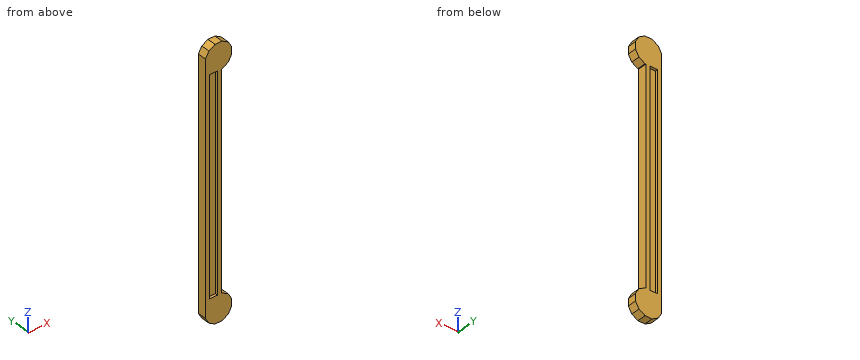
from build123d import *

# Parameters (mm, degrees)
BOSS_EXTRUDE1_DEPTH = 22
CUT_EXTRUDE1_DEPTH  = 635.24127901
SKETCH3_W           = 20
SKETCH3_H           = 534
CUT_EXTRUDE2_DEPTH  = 6.5
SKETCH4_W           = 20
SKETCH4_H           = 534
CUT_EXTRUDE3_DEPTH  = 6.5


with BuildPart() as part:
    # Sketch1 → Boss-Extrude1 (new body)
    with BuildSketch(Plane(origin=(0, 11, 0), x_dir=(1, 0, 0), z_dir=(0, 1, 0))):
        Polygon((24.15767665, 24.15767665), (8.84232335, 33), (-8.84232335, 33), (-24.15767665, 24.15767665), (-33, 8.84232335), (-33, -608.84232335), (-24.15767665, -624.15767665), (-8.84232335, -633), (8.84232335, -633), (24.15767665, -624.15767665), (33, -608.84232335), (33, 8.84232335), align=None)
    extrude(amount=-BOSS_EXTRUDE1_DEPTH)

    # Sketch2 → Cut-Extrude1 (cut, through all)
    with BuildSketch(Plane.XZ.offset(11)):
        Polygon((33, 8.84232335), (33, 591.15767665), (24.15767665, 575.84232335), (8.84232335, 567), (7, 567), (7, 33), (8.84232335, 33), (24.15767665, 24.15767665), align=None)
    extrude(amount=-CUT_EXTRUDE1_DEPTH, mode=Mode.SUBTRACT)

    # Sketch3 → Cut-Extrude2 (cut)
    with BuildSketch(Plane.XZ.offset(11)):
        with Locations((-13, 300)):
            Rectangle(SKETCH3_W, SKETCH3_H)
    extrude(amount=-CUT_EXTRUDE2_DEPTH, mode=Mode.SUBTRACT)

    # Sketch4 → Cut-Extrude3 (cut)
    with BuildSketch(Plane(origin=(0, 11, 0), x_dir=(-1, 0, 0), z_dir=(0, 1, 0))):
        with Locations((13, 300)):
            Rectangle(SKETCH4_W, SKETCH4_H)
    extrude(amount=-CUT_EXTRUDE3_DEPTH, mode=Mode.SUBTRACT)


solid = part.part
Read the model definition and answer for the solid it produces. Units are mm, in the model's axes. Round coordinates to 2 decimals unless told otherwise and drop trailing zeros. Order: outer loops, then holes, each group sorted by start corner. A loop starts at its lowest first (then second) coordinate and runs counter-clockwise, first axis right, second up.
1) Straight lines are drawn through the part: L1, parallel to X at y = -5.75, z = 401.5; L2, parallel to Z at x = -4, y = 5.25; L3, parallel to X at y = 3, z = 200.5. For each, find the intervals that lie inside material, in ascending order.
2) The part is cut by section B-B on x = 17. Write down the section's boundary in (y, z), plus the area to 3 significant figures.
3) The part is cut by section A-A on z = 105.5. Write down the section's boundary in (x, y), plus the area to 3 significant figures.
4) Flat-ended cylindrical pins translate along their axes: pin 1 (1 mm diameter, centred on x = 11, y = 2, fed in from -Z); pin 2 (4 mm diameter, centred on y = -6, z = 123, fed in from +X); pin 3 (2 mm diameter, centred on x = -16, y = 7.5, fed in from +Z). Find the tip coordinate at first contact, or state that the pin passes through.
Resolved:
1. L1: x = -33 to -23, -3 to 7
1. L2: z = -33 to 33, 567 to 633
1. L3: x = -33 to 7
2. outline: (-11, -28.29) - (11, -28.29) - (11, 28.29) - (-11, 28.29) - close; (-11, 571.71) - (11, 571.71) - (11, 628.29) - (-11, 628.29) - close
2. area: 2,490 mm2
3. outline: (-33, -11) - (-23, -11) - (-23, -4.5) - (-3, -4.5) - (-3, -11) - (7, -11) - (7, 11) - (-3, 11) - (-3, 4.5) - (-23, 4.5) - (-23, 11) - (-33, 11) - close
3. area: 620 mm2
4. pin 1: stops at z = -32.04
4. pin 2: stops at x = 7
4. pin 3: stops at z = 629.44
